Design review of the part built by this model. Coordinates are the model's own, in mm. A direction names the side the tool comes from. Give positions to 0.01 mm unless a question says otherwise; leave off trailing zeros. Write each loop counter-clockwise with the first axis right and the second up, starting at its lowest first coordinate (ties: lowest second). Pieces come first, ordered by that corner, then holes. Notation, with made-up numbers: M 84.25,32 L 125.25,32 A23 cw 125.25,46 Z; hole C -14,63.25 d8. An arc over 180 degrees is marked long. Answer in a Markdown table with one row per item.
```python
from build123d import *

# Parameters (mm, degrees)
F0_R     = 33.573471
F1_DEPTH = 25.4
F2_W     = 30.792393
F2_H     = 28.740146
F3_DEPTH = 25.4
F5_W     = 20.462201
F5_H     = 18.77485
F6_DEPTH = 25.4
F7_W     = 14.035523
F7_H     = 30.486682
F8_DEPTH = 25.4


with BuildPart() as f1:
    # F0 (on Top) → F1 (new body)
    with BuildSketch(Plane.XY):
        with Locations((0, 33.573471)):
            Circle(F0_R)
    extrude(amount=F1_DEPTH)

    # F5 (on face) → F6 (cut)
    with BuildSketch(Plane.XY.offset(25.4)):
        with Locations((0.784219, 34.929999)):
            Rectangle(F5_W, F5_H)
    extrude(amount=-F6_DEPTH, mode=Mode.SUBTRACT)

    # F7 (on face) → F8 (cut)
    with BuildSketch(Plane.XY.offset(25.4)):
        with Locations((1.928251, 10.299233)):
            Rectangle(F7_W, F7_H)
    extrude(amount=-F8_DEPTH, mode=Mode.SUBTRACT)


with BuildPart() as f3:
    # F2 (on Top) → F3 (new body)
    with BuildSketch(Plane.XY):
        with Locations((-49.557659, -41.295018)):
            Rectangle(F2_W, F2_H)
    extrude(amount=F3_DEPTH)


solid = f1.part
```
1) Add section C-C (z = 21.25). Write out the cut boundary in (x, y), and give its area (3 significant figures).
Geometry says:
| item | result |
|---|---|
| outline | M -9.45,25.54 L -9.45,44.32 L 11.02,44.32 L 11.02,25.54 L 8.95,25.54 L 8.95,1.21 A33.57 ccw long -5.09,0.39 L -5.09,25.54 Z |
| area | 2,800 mm^2 |
2) Add section A-A (x = -7). Write out the cut boundary in (y, z), and give its area (3 significant figures).
Geometry says:
| item | result |
|---|---|
| outline | M 0.74,0 L 25.54,0 L 25.54,25.4 L 0.74,25.4 Z; M 44.32,0 L 66.41,0 L 66.41,25.4 L 44.32,25.4 Z |
| area | 1,190 mm^2 |
3) Insertion check: P1, Ø3.5, axis at x = -7, z = 9, coming from the +Y side; P2, Ø5, axis at x = -17, z = 18.5, coming from the -Y side; P3, Ø9.5, axis at y = 34.5, z = 17, coming from the -X side. Each pin has a flat end and moves straight along its axis. Give the tip position at first contact, or say it passes through.
Geometry says:
| item | result |
|---|---|
| P1 | y = 66.73 |
| P2 | y = 3.29 |
| P3 | x = -33.57 |
4) Add section D-D (x = 0). Write out the cut boundary in (y, z).
Geometry says:
| item | result |
|---|---|
| outline | M 44.32,0 L 67.15,0 L 67.15,25.4 L 44.32,25.4 Z |
5) To check wall thickness, follow probe 1 along X at (y, z) = (34, 12); probe 2 along X at (y, z) = (44, 13.25); probe 3 along Y at (x, z) = (-6, 21.25). State the ranges of each line that lie inside material, in increasing order. Write a range as [from, to].
Geometry says:
| item | result |
|---|---|
| probe 1 | [-33.57, -9.45], [11.02, 33.57] |
| probe 2 | [-31.91, -9.45], [11.02, 31.91] |
| probe 3 | [0.54, 25.54], [44.32, 66.61] |
6) Add section B-B (y = 14.5). Write out the cut boundary in (x, z).
Geometry says:
| item | result |
|---|---|
| outline | M -27.63,0 L -5.09,0 L -5.09,25.4 L -27.63,25.4 Z; M 8.95,0 L 27.63,0 L 27.63,25.4 L 8.95,25.4 Z |
7) The part is to be moulded in two halves that separate along Y. For faces 1 (the face through (-9.447, 35, 13)), 2 (the face through (-5.09, 13, 13)), 3 (the face through (-0.6, 67.14, 12.52)), say which applies: released by +Y, released by -Y, zero draft, split by the parting line, or undercut.
Geometry says:
| item | result |
|---|---|
| face 1 | undercut |
| face 2 | zero draft |
| face 3 | split by the parting line |
8) For faces 4 (the face through (11.015, 35, 13)), 5 (the face through (0, 49, 0)), 6 (the face through (8.946, 13, 13)), list the 3-axis set-ups (+Z, -Z, +X, -X, +Y, -Y) from which the entire face can be reached by the end or side of a thin tool; tool diameter is ignored.
Geometry says:
| item | result |
|---|---|
| face 4 | +Z, -Z |
| face 5 | -Z, +X, -X, +Y, -Y |
| face 6 | +Z, -Z, -Y |
